Check sheet for the modelled part. Datum: model origin and axes. Units: mm. A direction names the side the tool comes from. Round coordinates to 2 decimals unless told otherwise and drop trailing zeros. Loops run counter-clockwise (first coordinate to the right, second up) from the corner with the lowest first, then second, coordinate; pieces in that order, holes last. Notation, with made-up numbers: M -37,53.5 L -12,53.5 A35 ccw -12,88.5 Z; hole C 17,42 d9. An arc over 180 degrees is marked long. Write item = value, one per line. Start each with the question number.
(1) Cross-section at B-B on x = 0. Record the boundary of the cut face in (y, z), plus the area to 3 significant figures.
(2) Go/stop test with flat-tipped pins: P1, Ø0.6, axis at x = 74.5, y = 1.5, coming from the +Z side; P2, Ø0.6, axis at x = -11, y = 1, coming from the -Z side; P3, Ø1, axis at y = 1, z = 19.5, coming from the +X side. Record where each tip stops, or that it passes through.
(3) Scan lines: L1, parallel to X at y = 1.1, z = 0; L2, parallel to X at y = 0.2, z = 6.5; L3, parallel to Z at x = -62, y = 0.65 (3 decimals). Record each from-to range of solid material in increasing order. Write a range as from..to.
(4) Cross-section at D-D on z = 61. Record the boundary of the cut face in (x, y), plus the area to 3 significant figures.
(5) Mould release check, pull along Z, two halves, no side actions. Record for faces 5 (the face through (-1, 2, 24)), 6 (the face through (-39.701, 0.986, 71.768)), 7 (the face through (-74.161, 0.986, 35.538)): pulls with the +Z half, pulls with the -Z half, needs draft (parallel to the pull), parting line crosses it, or undercut.
(6) Set-up check for faces 1 (the face through (-81.4, 1, -13.5)), 2 (the face through (73.993, 0.986, 35.38)), 3 (the face through (-58.356, 0.986, -57.882)), 4 (the face through (39.869, 0.986, 71.926)): record each of +Z, -Z, +X, -X, +Y, -Y from which the full face is reachable in a straight line by a thin tool's end or side.
(7) Cross-section at A-A on z = 13.5. Record the boundary of the cut face in (x, y).
(8) Cross-section at C-C on x = 37. Record the boundary of the cut face in (y, z).
from build123d import *

# Parameters (mm, degrees)
SKETCH1_R           = 10
BOSS_EXTRUDE1_DEPTH = 2


with BuildPart() as part:
    # Sketch1 → Boss-Extrude1 (new body)
    with BuildSketch(Plane(origin=(0, 0, 0), x_dir=(1, 0, 0), z_dir=(0, 1, 0))):
        with BuildLine():
            Line((74.750839635, 9.397976908), (62.630621153, 31.263481795))
            Line((62.630621153, 31.263481795), (50.510402672, 53.128986682))
            Line((50.510402672, 53.128986682), (65.676291813, 61.535556337))
            ThreePointArc((65.676291813, 61.535556337), (55.986333501, 70.466520143), (45.096073772, 77.886739118))
            Line((45.096073772, 77.886739118), (41, 61.886739118))
            Line((41, 61.886739118), (0, 61.886739118))
            Line((0, 61.886739118), (-41, 61.886739118))
            Line((-41, 61.886739118), (-45.096073772, 77.886739118))
            ThreePointArc((-45.096073772, 77.886739118), (-55.882783617, 70.548667565), (-65.495262312, 61.728199509))
            Line((-65.495262312, 61.728199509), (-51.013470384, 53.925622849))
            Line((-51.013470384, 53.925622849), (-62.871489624, 31.916820526))
            Line((-62.871489624, 31.916820526), (-74.729508865, 9.908018203))
            Line((-74.729508865, 9.908018203), (-88.333788079, 17.237803909))
            ThreePointArc((-88.333788079, 17.237803909), (-89.109620692, -12.628360942), (-80.06590623, -41.102927627))
            Line((-80.06590623, -41.102927627), (-68.088543882, -29.815267766))
            Line((-68.088543882, -29.815267766), (-50.942469943, -48.009007032))
            Line((-50.942469943, -48.009007032), (-33.796396003, -66.202746297))
            Line((-33.796396003, -66.202746297), (-45.773758351, -77.490406158))
            ThreePointArc((-45.773758351, -77.490406158), (0, -90), (45.773758351, -77.490406158))
            Line((45.773758351, -77.490406158), (33.796396003, -66.202746297))
            Line((33.796396003, -66.202746297), (50.942469943, -48.009007032))
            Line((50.942469943, -48.009007032), (68.088543882, -29.815267766))
            Line((68.088543882, -29.815267766), (80.06590623, -41.102927627))
            ThreePointArc((80.06590623, -41.102927627), (87.481231018, -21.143183763), (90, 0))
            ThreePointArc((90, 0), (89.596114425, 8.516823346), (88.388082669, 16.957206202))
            Line((88.388082669, 16.957206202), (74.750839635, 9.397976908))
        make_face()
        Polygon((-68, 5), (-68, -4), (-40, -4), (-40, -16), (-68, -16), (-68, -25), (-81, -25), (-81, 5), align=None, mode=Mode.SUBTRACT)
        Polygon((-15, -63), (-6, -63), (-6, -35), (6, -35), (6, -63), (15, -63), (15, -76), (-15, -76), align=None, mode=Mode.SUBTRACT)
        Polygon((68, -25), (68, -16), (40, -16), (40, -4), (67.990906131, -4), (67.990906131, 5), (80.990906131, 5), (80.990906131, -25), align=None, mode=Mode.SUBTRACT)
        Polygon((15, 43), (6, 43), (6, 15), (-6, 15), (-6, 42), (-15, 42), (-15, 55), (15, 55), align=None, mode=Mode.SUBTRACT)
        with Locations(Location((0, 0, 0), (0, 0, 270))):
            Circle(SKETCH1_R, mode=Mode.SUBTRACT)
    extrude(amount=BOSS_EXTRUDE1_DEPTH)


solid = part.part
Result:
q1.outline = M 0,-61.89 L 2,-61.89 L 2,-55 L 0,-55 Z; M 0,-15 L 2,-15 L 2,-10 L 0,-10 Z; M 0,10 L 2,10 L 2,35 L 0,35 Z; M 0,76 L 2,76 L 2,90 L 0,90 Z
q1.area = 102 mm^2
q2.P1 = 36.14
q2.P2 = -61.89
q2.P3 = 87.97
q3.L1 = -90..-81, -68..-10, 10..67.99, 80.99..90
q3.L2 = -89.76..-81, -40..-7.6, 7.6..40, 80.99..89.76
q3.L3 = -65.238..-59.845, -33.534..4, 16..36.276
q4.outline = M -38.7,0 L -6,0 L -6,2 L -38.7,2 Z; M 6,0 L 38.7,0 L 38.7,2 L 6,2 Z
q4.area = 131 mm^2
q5.face_5 = needs draft
q5.face_6 = undercut
q5.face_7 = pulls with the +Z half
q6.face_1 = -Z, +Y, -Y
q6.face_2 = +Z, +Y, -Y
q6.face_3 = -X, +Y, -Y
q6.face_4 = +X, +Y, -Y
q7.outline = M -88.98,0 L -81,0 L -81,2 L -88.98,2 Z; M -40,0 L 40,0 L 40,2 L -40,2 Z; M 80.99,0 L 88.98,0 L 88.98,2 L 80.99,2 Z
q8.outline = M 0,-61.89 L 2,-61.89 L 2,62.8 L 0,62.8 Z; M 0,69.22 L 2,69.22 L 2,82.04 L 0,82.04 Z
